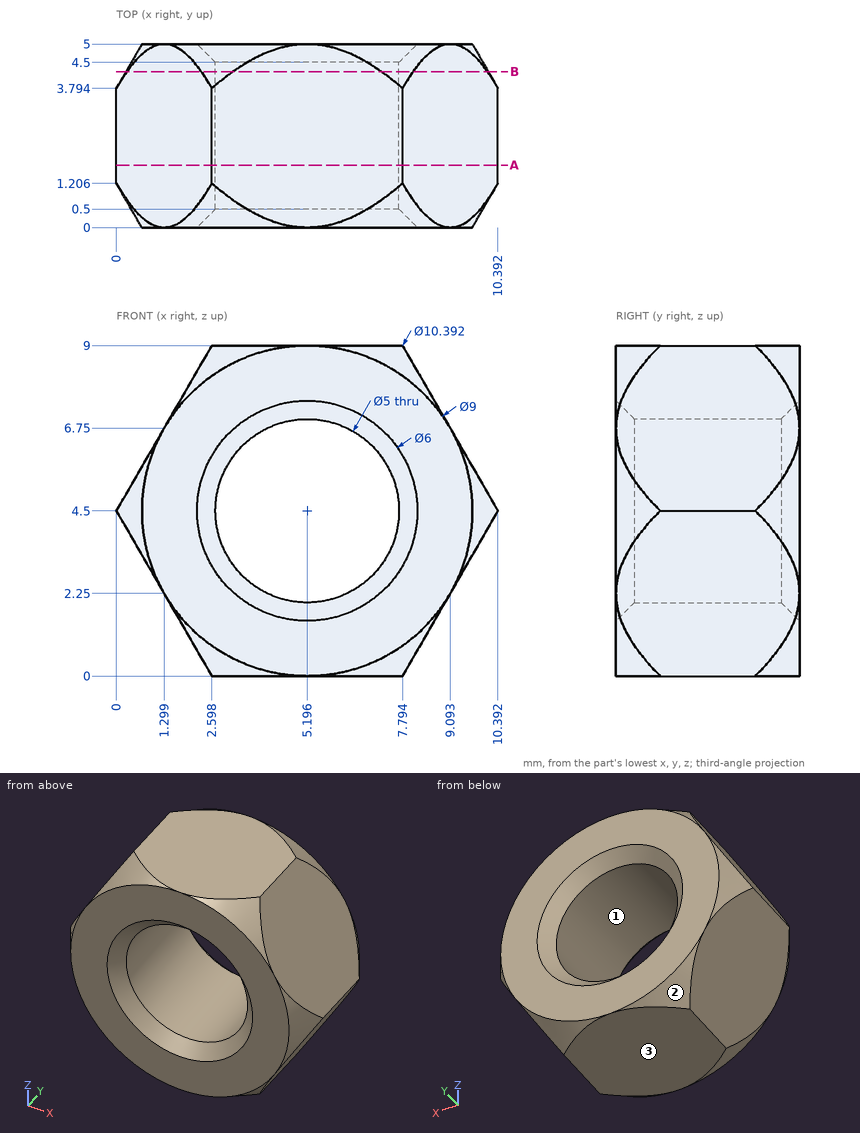
Answer from the drawing. Dimensions are ordinates in mm from the lowest x, y and z of the part. Round coordinates to 2 decimals unless told otherwise and drop trailing zeros. Write each loop counter-clockwise with the first axis right and the second up, starting at its lowest first coordinate (ties: lowest second). Pieces come first, ordered by that corner, then holes. Notation, with made-up numbers: (35.5, 58) -> (59.5, 58) arc R24 ccw to (59.5, 71) -> close; hole circle Ø1 at (76.25, -40). An arc over 180 degrees is marked (long way). Answer in a Markdown table with one row per item. Add a question column.
1) Given P1, Ø3, axis at x = 5.2, z = 4.5, coming from the +Y side, flat-ended and moving along its own axis, determine where the tip first touches the part or whether it passes through.
2) Determine the mould class of the marked faces 1, 2 and 3 for opening direction X: pulls with the +X half, pulls with the -X half, needs draft (parallel to the pull), parting line crosses it, or undercut.
3) Find section B-B, the plane y = 4.25. Determine the outline of the cut face in (x, z) (1 decimal).
4) Find section A-A, the plane y = 1.7. Determine the outline of the cut face in (x, z), and give its area (3 significant figures).
5) Consider line 1 (Z direction, x = 7, y = 1.9); line 2 (X direction, y = 2.6, z = 4.25) (1 decimal); line 3 (X direction, y = 1.25, z = 5) (1 decimal). Determine where each line is inside the solid, lowest interval first.
Findings below:
| question | item | result |
|---|---|---|
| 1 | P1 | through |
| 2 | face 1 | undercut |
| 2 | face 2 | pulls with the -X half |
| 2 | face 3 | needs draft |
| 3 | outline | (0.3, 4) -> (2.3, 0.5) arc R4.9 ccw to (3.2, 0) -> (7.2, 0) arc R4.9 ccw to (8.1, 0.5) -> (10.1, 4) arc R4.9 ccw to (10.1, 5) -> (8.1, 8.5) arc R4.9 ccw to (7.2, 9) -> (3.2, 9) arc R4.9 ccw to (2.3, 8.5) -> (0.3, 5) arc R4.9 ccw to start; hole circle Ø5 at (5.2, 4.5) |
| 4 | outline | (0, 4.5) -> (2.6, 0) -> (7.79, 0) -> (10.39, 4.5) -> (7.79, 9) -> (2.6, 9) -> close; hole circle Ø5 at (5.2, 4.5) |
| 4 | area | 50.5 mm² |
| 5 | line 1 | 0 to 2.77, 6.23 to 9 |
| 5 | line 2 | 0.1 to 2.7, 7.7 to 10.2 |
| 5 | line 3 | 0.3 to 2.7, 7.6 to 10.1 |
